Source: CAD feature listing. Evaluate the final solid. Frame: model axes, mm. A direction names the side the tool comes from. Round coordinates to 2 decimals unless told otherwise and drop trailing zeros. Loops run counter-clockwise (first coordinate to the right, second up) from the corner with the lowest first, then second, coordinate; pieces in that order, holes last. Notation, with made-up numbers: M 20.25,18 L 75.25,18 A31 ccw 75.25,46 Z; hole C 44,65.25 d2. An arc over 180 degrees is marked long. One line per item, written item: value.
from build123d import *

# Parameters (mm, degrees)
SKETCH1_W             = 38.1
SKETCH1_H             = 38.1
SKETCH1_W_2           = 34.925
SKETCH1_H_2           = 34.925
BOSS_EXTRUDE1_DEPTH   = 78.58125
SKETCH2_W             = 38.1
SKETCH2_H             = 38.1
SKETCH2_W_2           = 30.1625
SKETCH2_H_2           = 30.1625
BOSS_EXTRUDE2_DEPTH   = 1.5875
SKETCH3_W             = 1.5875
SKETCH3_H             = 6.35
BOSS_EXTRUDE3_DEPTH   = 12.7
SKETCH3_W_2           = 6.35
SKETCH3_H_2           = 1.5875
BOSS_EXTRUDE3_2_DEPTH = 12.7
BOSS_EXTRUDE3_3_DEPTH = 12.7
BOSS_EXTRUDE3_4_DEPTH = 12.7
SKETCH4_R             = 1.5875
CUT_EXTRUDE3_DEPTH    = 50.8
SKETCH5_R             = 1.5875
CUT_EXTRUDE4_DEPTH    = 50.8
SKETCH6_W             = 6.35
SKETCH6_H             = 1.5875
SKETCH6_W_2           = 1.5875
SKETCH6_H_2           = 6.35
BOSS_EXTRUDE4_DEPTH   = 3.175
FILLET3_R             = 0.79375
FILLET4_R             = 3.175
SKETCH7_W             = 38.354
SKETCH7_H             = 38.354
CUT_EXTRUDE5_DEPTH    = 25.4


with BuildPart() as part:
    # Sketch1 → Boss-Extrude1 (new body)
    with BuildSketch(Plane(origin=(0, 0, 0), x_dir=(1, 0, 0), z_dir=(0, 1, 0))):
        Rectangle(SKETCH1_W, SKETCH1_H)
        Rectangle(SKETCH1_W_2, SKETCH1_H_2, mode=Mode.SUBTRACT)
    extrude(amount=BOSS_EXTRUDE1_DEPTH)

    # Sketch2 → Boss-Extrude2 (add)
    with BuildSketch(Plane(origin=(0, 78.58125, 0), x_dir=(1, 0, 0), z_dir=(0, 1, 0))):
        Rectangle(SKETCH2_W, SKETCH2_H)
        Rectangle(SKETCH2_W_2, SKETCH2_H_2, mode=Mode.SUBTRACT)
    extrude(amount=BOSS_EXTRUDE2_DEPTH)



with BuildPart() as body_2:
    # Sketch3 → Boss-Extrude3 (new body)
    with BuildSketch(Plane.XZ):
        with Locations((-19.84375, 0)):
            Rectangle(SKETCH3_W, SKETCH3_H)
    extrude(amount=BOSS_EXTRUDE3_DEPTH)


with BuildPart() as body_3:
    # Sketch3 → Boss-Extrude3 2 (new body)
    with BuildSketch(Plane.XZ):
        with Locations((0, 19.84375)):
            Rectangle(SKETCH3_W_2, SKETCH3_H_2)
    extrude(amount=BOSS_EXTRUDE3_2_DEPTH)


with BuildPart() as body_4:
    # Sketch3 → Boss-Extrude3 3 (new body)
    with BuildSketch(Plane.XZ):
        with Locations((19.84375, 0)):
            Rectangle(SKETCH3_W, SKETCH3_H)
    extrude(amount=BOSS_EXTRUDE3_3_DEPTH)


with BuildPart() as body_5:
    # Sketch3 → Boss-Extrude3 4 (new body)
    with BuildSketch(Plane.XZ):
        with Locations((0, -19.84375)):
            Rectangle(SKETCH3_W_2, SKETCH3_H_2)
    extrude(amount=BOSS_EXTRUDE3_4_DEPTH)


with BuildPart() as cut_extrude3_tool:
    # Sketch4 → Cut-Extrude3 (new body)
    with BuildSketch(Plane.XY.offset(20.6375)):
        with Locations((0, -9.017)):
            Circle(SKETCH4_R)
    extrude(amount=-CUT_EXTRUDE3_DEPTH)


with BuildPart() as body_3_1:
    add(body_3.part)

    # Cut-Extrude3: cut by cut_extrude3_tool
    add(cut_extrude3_tool.part, mode=Mode.SUBTRACT)


with BuildPart() as body_5_1:
    add(body_5.part)

    # Cut-Extrude3: cut by cut_extrude3_tool
    add(cut_extrude3_tool.part, mode=Mode.SUBTRACT)


with BuildPart() as cut_extrude4_tool:
    # Sketch5 → Cut-Extrude4 (new body)
    with BuildSketch(Plane(origin=(20.6375, 0, 0), x_dir=(0, 0, -1), z_dir=(1, 0, 0))):
        with Locations((0, -9.017)):
            Circle(SKETCH5_R)
    extrude(amount=-CUT_EXTRUDE4_DEPTH)


with BuildPart() as body_2_1:
    add(body_2.part)

    # Cut-Extrude4: cut by cut_extrude4_tool
    add(cut_extrude4_tool.part, mode=Mode.SUBTRACT)


with BuildPart() as body_4_1:
    add(body_4.part)

    # Cut-Extrude4: cut by cut_extrude4_tool
    add(cut_extrude4_tool.part, mode=Mode.SUBTRACT)


with BuildPart() as part_1:
    add(part.part)

    add(body_2_1.part)  # Boss-Extrude4 merges body 2

    add(body_3_1.part)  # Boss-Extrude4 merges body 3

    add(body_4_1.part)  # Boss-Extrude4 merges body 4

    add(body_5_1.part)  # Boss-Extrude4 merges body 5
    # Sketch6 → Boss-Extrude4 (add)
    with BuildSketch(Plane(origin=(0, 0, 0), x_dir=(1, 0, 0), z_dir=(0, 1, 0))):
        with Locations((0, 19.84375)):
            Rectangle(SKETCH6_W, SKETCH6_H)
        with Locations((19.84375, 0)):
            Rectangle(SKETCH6_W_2, SKETCH6_H_2)
        with Locations((0, -19.84375)):
            Rectangle(SKETCH6_W, SKETCH6_H)
        with Locations((-19.84375, 0)):
            Rectangle(SKETCH6_W_2, SKETCH6_H_2)
    extrude(amount=BOSS_EXTRUDE4_DEPTH)

    # Fillet3
    fillet3_edges = [part_1.edges().sort_by_distance(p)[0] for p in [
        (-19.05, 3.175, 0),
        (0, 3.175, -19.05),
        (19.05, 3.175, 0),
        (0, 3.175, 19.05),
    ]]
    fillet(fillet3_edges, radius=FILLET3_R)
    fillet3_2_edges = [part_1.edges().sort_by_distance(p)[0] for p in [
        (-20.6375, 3.175, 0),
        (0, 3.175, -20.6375),
        (20.6375, 3.175, 0),
        (0, 3.175, 20.6375),
    ]]
    fillet(fillet3_2_edges, radius=FILLET3_R - 0.0001)  # a hair under: the kernel refuses the full size

    # Fillet4
    fillet4_edges = [part_1.edges().sort_by_distance(p)[0] for p in [
        (3.175, -12.7, -19.84375),
        (-3.175, -12.7, -19.84375),
        (19.84375, -12.7, -3.175),
        (19.84375, -12.7, 3.175),
        (3.175, -12.7, 19.84375),
        (-3.175, -12.7, 19.84375),
        (-19.84375, -12.7, 3.175),
        (-19.84375, -12.7, -3.175),
    ]]
    fillet(fillet4_edges, radius=FILLET4_R - 0.0001)  # a hair under: the kernel refuses the full size

    # Sketch7 → Cut-Extrude5 (cut)
    with BuildSketch(Plane.XZ):
        Rectangle(SKETCH7_W, SKETCH7_H)
    extrude(amount=CUT_EXTRUDE5_DEPTH, mode=Mode.SUBTRACT)


solid = part_1.part
1. Ray query, line 1 (Z direction, x = -0.5, y = 41); line 2 (Y direction, x = 20, z = 0). Return the intervals inside material, ascending. Write a range as [from, to].
Report:
line 1: z = [-19.05, -17.46], [17.46, 19.05]
line 2: y = [-12.7, -10.6], [-7.43, 3.16]
2. Pin query (flat end, axial travel): pin 1 (1.3 mm diameter, centred on y = 79.5, z = -5.5, fed in from -X); pin 2 (2 mm diameter, centred on x = -13.5, y = 58, fed in from +Z); pin 3 (1.3 mm diameter, centred on y = 79, z = 2.5, fed in from +X). Return the tip coordinate at first contact, or that it passes through.
Report:
pin 1: stops at x = -19.05
pin 2: stops at z = 19.05
pin 3: stops at x = 19.05
3. Section query C-C (x = -13). Return the cut outline in (y, z).
Report:
outline: M 0,-19.05 L 80.17,-19.05 L 80.17,-15.08 L 78.58,-15.08 L 78.58,-17.46 L 0,-17.46 Z; M 0,17.46 L 78.58,17.46 L 78.58,15.08 L 80.17,15.08 L 80.17,19.05 L 0,19.05 Z
4. Reachability of faces 1 (the face through (-19.897, -11.745, -2.27)), 2 (the face through (15.3, 78.581, -0.2)) from +Z, -Z, +X, -X, +Y, -Y: full face, straight path, thin tool, end or side. Return the list, or none.
Report:
face 1: -Z, +X, -X, -Y
face 2: -Y
5. Section query A-A (y = 13.5). Return the cut outline in (x, z).
Report:
outline: M -19.05,-19.05 L 19.05,-19.05 L 19.05,19.05 L -19.05,19.05 Z; hole M -17.46,-17.46 L 17.46,-17.46 L 17.46,17.46 L -17.46,17.46 Z
6. Section query B-B (z = 6.5). Return the cut outline in (x, y).
Report:
outline: M -19.05,0 L -17.46,0 L -17.46,78.58 L -15.08,78.58 L -15.08,80.17 L -19.05,80.17 Z; M 15.08,78.58 L 17.46,78.58 L 17.46,0 L 19.05,0 L 19.05,80.17 L 15.08,80.17 Z
7. Section query D-D (x = 16.5). Return the cut outline in (y, z).
Report:
outline: M 0,-19.05 L 80.17,-19.05 L 80.17,19.05 L 0,19.05 L 0,17.46 L 78.58,17.46 L 78.58,-17.46 L 0,-17.46 Z
8. Pull-direction query (Z, two-part tool) for faces 3 (the face through (0, -6, 19.177)), 4 (the face through (0, -6, -19.177)), 5 (the face through (19.917, -11.745, -2.27)), 6 (the face through (-19.177, -6, 0)); classes: released by +Z, released by -Z, zero draft, split by the parting line, or undercut.
Report:
face 3: undercut
face 4: undercut
face 5: released by -Z
face 6: zero draft
